Autodesk Inventor part; units mm, degrees
ref_plane "YZ Plane" through (0, 0, 0) normal (1, 0, 0) x (0, 1, 0)
ref_plane "XZ Plane" through (0, 0, 0) normal (0, 1, 0) x (-1, 0, 0)
ref_plane "XY Plane" through (0, 0, 0) normal (0, 0, 1) x (1, 0, 0)
sketch "Sketch2" plane through (0, 0, 0) normal (1, 0, 0) x (0, 1, 0)
  line L0 (17.5, 10.75) -> (-17.5, 10.75)
  line L1 (-17.5, 10.75) -> (-17.5, -28.75)
  line L2 (-17.5, -28.75) -> (17.5, -28.75)
  line L3 (17.5, -28.75) -> (17.5, 10.75)
  line L4 (17.5, 10.75) -> (-17.5, -28.75) construction
  line L5 (-17.5, 10.75) -> (17.5, -28.75) construction
  line L6 (-55, -9.75) -> (55, -9.75)
  line L7 (55, -9.75) -> (55, -15.4999)
  line L8 (55, -15.4999) -> (-55, -15.4999)
  line L9 (-55, -15.4999) -> (-55, -9.75)
  line L10 (-55, -9.75) -> (55, -15.4999) construction
  line L11 (55, -9.75) -> (-55, -15.4999) construction
  line L12 (46, -9.75) -> (46, -15.4999)
  line L13 (0, 65.9057) -> (0, -65.9057)
  circle A0 centre (75.7124, 0) radius 25
  line L14 (0, 0) -> (82.4805, 0) construction
  line L15 (-55, 9.75) -> (55, 9.75)
  line L16 (55, 9.75) -> (55, 15.4999)
  line L17 (55, 15.4999) -> (-55, 15.4999)
  line L18 (-55, 15.4999) -> (-55, 9.75)
  line L19 (46, 9.75) -> (46, 15.4999)
  line L20 (0, 24.9999) -> (49, 24.9999)
  line L21 (49, 24.9999) -> (49, 15.4999)
  line L22 (0, 30.9999) -> (12.5, 30.9999)
  line L23 (12.5, 30.9999) -> (12.5, 24.9999)
  line L24 (0, -28.75) -> (5, -28.75)
  line L25 (5, -28.75) -> (5, -46.25)
  line L26 (5, -46.25) -> (0, -46.25)
  line L27 (0, -46.25) -> (0, -28.75)
  line L28 (0, 30.9999) -> (5, 30.9999)
  line L29 (5, 30.9999) -> (5, 46.7999)
  line L30 (5, 46.7999) -> (0, 46.7999)
  line L31 (0, 46.7999) -> (0, 30.9999)
  point P0 (0, -9)
  point P1 (0, -9)
  point P2 (0, -12.625)
  point P3 (0, -12.625)
  point P4 (0, -12.625)
  point P5 (0, -9)
  point P6 (55, -13.9999)
  point P7 (0, 12.625)
  point P8 (55, 13.9999)
  point P9 (55, 13.9999)
  point P10 (0, -30)
  point P11 (17.5, -15.4999)
  point P12 (0, -46.25)
  point P13 (5, -28.75)
  point P14 (0, 46.7999)
  point P15 (5, 30.9999)
  point P16 (99.7681, -6.8058)
  point P17 (0, 10.75)
  point P18 (17.5, -9.75)
  dimension "d0" = 35
  dimension "d1" = 39.5
  dimension "d2" = 9
  dimension "d3" = 110
  dimension "d7" = 9
  dimension "d12" = 49
  dimension "d13" = 9.5
  dimension "d14" = 12.5
  dimension "d15" = 6
  dimension "d42" = 5
  dimension "d43" = 17.5
  dimension "d44" = 5
  dimension "d45" = 15.8
  dimension "d53" = 100
  dimension "d74" = 19
  dimension "d75" = 50
  dimension "d76" = 1.5
revolve "Revolution1" add sketch "Sketch2" angle 360 about axis through (0, 0, 65.9057) along (0, 0, -1) contours L3 L15 L13 L0 | L0 L13 L17 L19 L15 L3 | L15 A0 L6 L3 | L3 L6 L13 L15 | L13 L20 L21 L17 | L3 L8 L13 L6 | L19 L17 L16 A0 L15 | L13 L22 L23 L20 | L3 L2 L13 L8 | L6 A0 L7 L8 L12 | L15 L16 A0 L7 L6 | A0 L16 L15 | L13 L30 L29 L22 | L6 L7 A0 | L2 L25 L26 L13
sketch "Sketch4" plane through (0, 0, 24.9999) normal (0, 0, 1) x (1, 0, 0)
  circle A0 centre (32.15, 0) radius 6.15
  circle A1 centre (32.15, 0) radius 2.15
  circle A2 centre (0, 0) radius 49
  circle A3 centre (0, 0) radius 49
  line L0 (26, 14.6294) -> (26, -8.2066)
  circle A4 centre (0, 0) radius 36
  circle A5 centre (0, 0) radius 15
  line L1 (-8.8861, 39.8) -> (0.1206, 45)
  line L2 (0.1206, 45) -> (9.8706, 28.1125)
  line L3 (9.8706, 28.1125) -> (0.8639, 22.9125)
  line L4 (0.8639, 22.9125) -> (-8.8861, 39.8)
  line L5 (-8.8861, 39.8) -> (9.8706, 28.1125) construction
  line L6 (0.1206, 45) -> (0.8639, 22.9125) construction
  line L7 (0, 0) -> (49, 0) construction
  circle A6 centre (0.4923, -33.9563) radius 12
  line L8 (0.5569, -29.2189) -> (-43.347, -0.503)
  line L9 (-43.347, -0.503) -> (-52.105, -13.8932)
  line L10 (-52.105, -13.8932) -> (-6.0762, -43.9989)
  line L11 (-4.0111, 31.3563) -> (-50.7764, 4.3563) construction
  point P0 (0, 0)
  point P1 (0.4923, 33.9563)
  point P2 (5.5667, 35.567)
  point P3 (35.6423, 5.0622)
  point P4 (35.6423, -5.0622)
  point P5 (-6.3647, 35.4329)
  point P6 (0.4923, 33.9563)
  point P7 (-6.7865, -24.4159)
  point P8 (-48.9, 3.1289)
  point P9 (-45.4855, -18.2228)
  point P10 (-48.3238, -8.1121)
  dimension "d55" = 24
  dimension "d24" = 12.3
  dimension "d25" = 4
  dimension "d26" = 23
  dimension "d29" = 72
  dimension "d30" = 30
  dimension "d31" = 10.4
  dimension "d32" = 19.5
  dimension "d33" = 60
  dimension "d34" = 98
  dimension "d35" = 45
  dimension "d54" = 46.4246
  dimension "d56" = 16
  dimension "d57" = 54
  dimension "d62" = 55
extrude "Extrusion1" add sketch "Sketch4" along normal blind 6 contours A0 A4 | A4 A0
extrude "Extrusion2" add sketch "Sketch4" along normal blind 1.5 contours A0 A4 L2 L1 L4 L8 L9 A2 L10 A6 | A6 A4 | A6 L10 A2 L9 L8 A4 picked at (0.1047, -39.1419)
extrude "Extrusion3" add sketch "Sketch4" along normal blind 2.5 contours A5
extrude "Extrusion4" add sketch "Sketch4" along normal blind 14.5 contours L2 L3 L4 A4 | A4 L4 L1 L2
sketch "Sketch3" plane through (0, 0, 30.9999) normal (0, 0, 1) x (1, 0, 0)
  point P0 (0, 0)
  point P1 (0, 0)
hole "Hole1" [suppressed]
chamfer "Chamfer1" distance 2 angle 45 2 edges at (0, -5, 46.7999) (0, -5, -46.25)
thread "Thread1"
thread "Thread2"
extrude "Extrusion5" add sketch "Sketch4" along normal blind 15 contours A6 A4 | A4 A6
extrude "Extrusion6" add sketch "Sketch4" along normal blind 20 contours A6 L10 A2 L9 L8 A4 | A4 L8 A6 | L10 L9 A2
sketch "Sketch5" plane through (9.8706, 28.1125, 39.4999) normal (0.866, 0.5, 0) x (0, 0, -1)
  line L0 (13, 19.5) -> (13, 8.6077)
  line L1 (13, 19.5) -> (0, 19.5)
  line L2 (0, 0) -> (0, 19.5)
  line L3 (14.5, 0) -> (0, 0)
  line L4 (14.5, 8.6077) -> (14.5, 0)
  line L5 (14.5, 8.6077) -> (13, 8.6077)
  circle A0 centre (7.5, 5.5) radius 4
  line L6 (3.5, 17.7174) -> (3.5, 4.9566) construction
  line L7 (3.5, 9.5) -> (10.4741, 9.5) construction
  line L8 (14.5, 0) -> (0, 0)
  line L9 (6.5, 0) -> (6.5, 5.5)
  line L10 (8.5, 5.5) -> (8.5, 0)
  line L11 (6.5, 5.5) -> (8.5, 5.5) construction
  point P0 (39.4999, -19.4108)
  point P1 (8.5, 2.75)
  point P2 (6.5, 2.75)
  point P3 (6.5, 1.627)
  point P4 (6.5, 0)
  point P5 (8.5, 1.627)
  dimension "d63" = 8
  dimension "d64" = 3.5
  dimension "d65" = 10
  dimension "d66" = 2
extrude "Extrusion7" cut sketch "Sketch5" against normal up to surface (10.4 mm away) contours L9 A0 L10 L3 | A0
extrude "Extrusion8" cut sketch "Sketch5" against normal through all contours L9 A0 L10 L3
thread "Thread3"
equation "\"d42\" = d44"
properties part number "FreeBackWheel" material "Rubber"
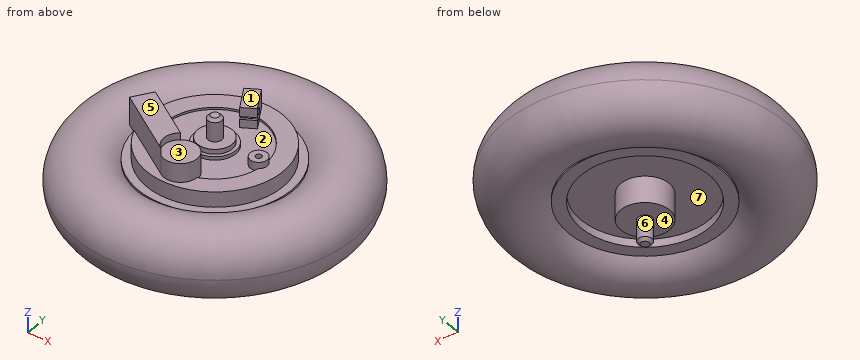
The listing builds one solid part. Answer for the finished solid, in the listing's coordinates (mm). Face numbers are marked on the shaded views. A direction names the side the tool comes from. Give positions to 0.01 mm unless a question says otherwise; leave off trailing zeros. Order: outer loops, then holes, each group sorted by start corner. A loop starts at its lowest first (then second) coordinate and runs counter-clockwise, first axis right, second up. Notation, with made-up numbers: M -6.5,63 L 27.5,63 A28 cw 27.5,81 Z; hole C -29,-3 d3. An arc over 180 degrees is marked long. Put each result on its own line as item: value. Start each with the question number.
Item 1: The part is cut by section A-A, the plane z = -21. Determine the outline of the cut face in (x, y).
Item 2: For a pull along X with two mould halves and no side action, classify the marked faces 5, 6 and 7 as +X half, -X half, draft (parallel to the pull), parting line (faces both ways), or undercut.
Item 3: Which of the six approach directions +Z, -Z, +X, -X, +Y, -Y give full straight-line access (tool end or side, diameter ignored) to the marked faces 1, 2, 3 and 4?
Item 4: Flat-ended cylindrical pins translate along their axes: P1, Ø3, axis at x = -1.5, z = 13, coming from the +Y side; P2, Ø3, axis at x = 60, y = 72.5, coming from the -Z side; P3, Ø5, axis at x = -19, z = 32.5, coming from the +Y side; P4, Ø24, axis at x = -2, y = 5.5, coming from the +Z side. Find the tip coordinate at first contact, or state that the pin passes through.
Item 5: The part is cut by section B-B, the plane z = -33. Determine the outline of the cut face in (x, y), and give its area (3 significant figures).
Item 6: The part is cut by section C-C, the plane z = -5. Determine the outline of the cut face in (x, y), and give its area (3 significant figures).
Item 7: Find the intervals of material crossed by line 1 along Y through (x, z) = (32, 28); line 2 along X through (y, z) = (9, -18.5); line 3 along X through (y, z) = (-36, -14.5), in increasing order.
Answer key:
1. outline: C 0,0 d178.55; C 0,0 d35; hole C 0,0 d124.3
2. face 5: draft
2. face 6: parting line
2. face 7: undercut
3. face 1: +Z, +X, -X, +Y
3. face 2: +Z
3. face 3: +Z, +X
3. face 4: -Z
4. P1: stops at y = 97.9
4. P2: stops at z = -18.43
4. P3: stops at y = -14.79
4. P4: stops at z = 46.8
5. outline: C 0,0 d10
5. area: 78.5 mm²
6. outline: C 0,0 d200.41
6. area: 31,500 mm²
7. line 1: y = -6.15 to -2.14, 2.14 to 6.15
7. line 2: x = -92.09 to -58.21, -15.01 to 15.01, 58.21 to 92.09
7. line 3: x = -89.08 to -42.04, -41.58 to -28.64, 28.64 to 41.58, 42.04 to 89.08
